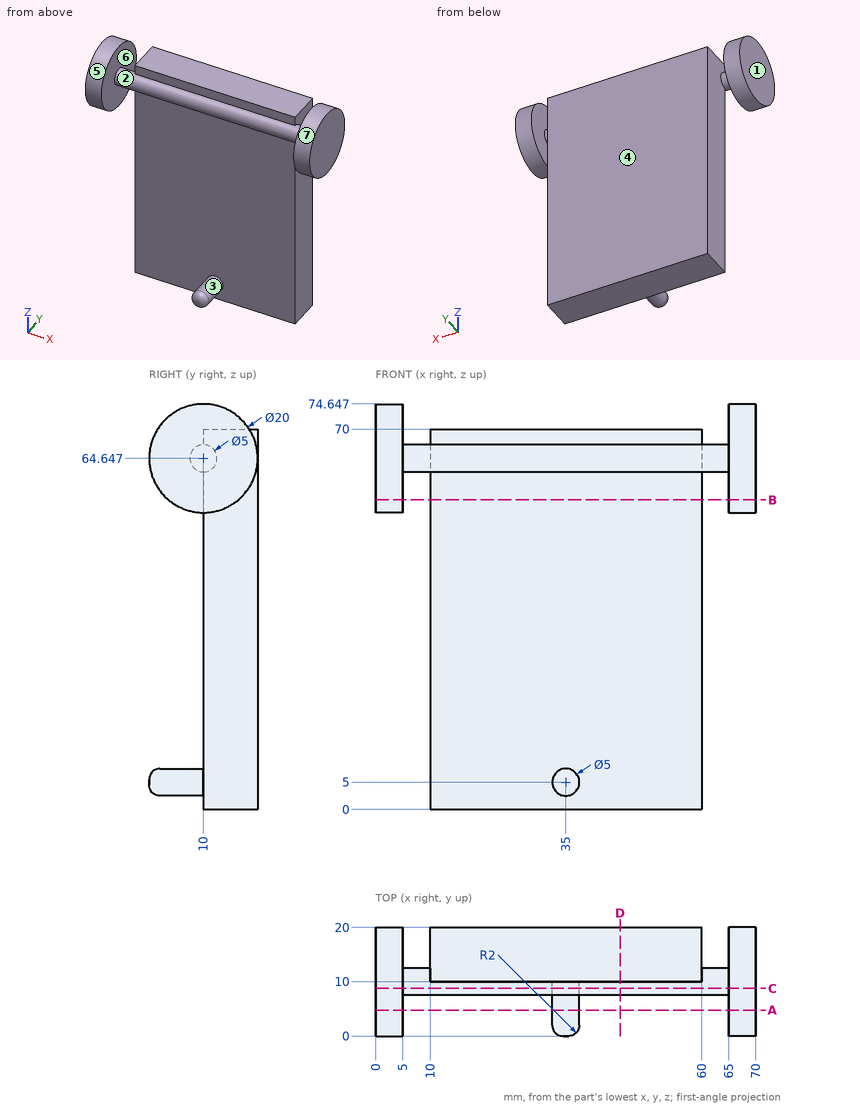
Geometry: see drawing. Coordinates: mm, zero at the bounding-box minimum. A direction names the side the tool comes from. Coordinates: 2 decimals unless noted, no trailing zeros. Order: outer loops, then holes, each group sorted by start corner. A loop starts at its lowest first (then second) coordinate and runs counter-clockwise, first axis right, second up. Notation, with made-up numbers: (38.5, 0.25) - (97.5, 0.25) arc R17 ccw to (97.5, 4.25) - close; hole circle Ø9 at (-35, 65). An arc over 180 degrees is marked (long way). Return JSON: item names as keys, results as strings.
Q1. First-contact query: pin 1 (0.9 mm diameter, centred on x = 44, z = 68.5, fed in from -Y); pin 2 (3 mm diameter, centred on y = 15, z = 34.5, fed in from +X); pin 3 (2 mm diameter, centred on x = 54.5, y = 9.5, fed in from +Z). Flat tips, straight axial feed; report the tip coordinate or a pass-through.
The answers:
{"pin 1": "stops at y = 10", "pin 2": "stops at x = 60", "pin 3": "stops at z = 70"}
Q2. Ray query, probe 1 along X at (y, z) = (13.5, 57); probe 2 along X at (y, z) = (13, 32.5); probe 3 along Y at (x, z) = (30, 64.5). Return the intervals inside material, ascending.
The answers:
{"probe 1": "x = 0 to 5, 10 to 60, 65 to 70", "probe 2": "x = 10 to 60", "probe 3": "y = 7.5 to 20"}
Q3. Cut plane C-C (y = 8.75). Return loops of the section in (x, z) (1 decimal), then the cut area to 3 significant figures.
The answers:
{"outline": "(0, 54.7) - (5, 54.7) - (5, 62.5) - (65, 62.5) - (65, 54.7) - (70, 54.7) - (70, 74.6) - (65, 74.6) - (65, 66.8) - (5, 66.8) - (5, 74.6) - (0, 74.6) - close; circle Ø5 at (35, 5)", "area": "478 mm2"}
Q4. Draft query along X for the marked faces 1, 2, 3 and 4. Return one class per face: +X half, -X half, draft (parallel to the pull), parting line (faces both ways), or undercut.
The answers:
{"face 1": "-X half", "face 2": "undercut", "face 3": "parting line", "face 4": "draft"}
Q5. Cut plane B-B (z = 57). Return loops of the section in (x, y), then the cut area to 3 significant figures.
The answers:
{"outline": "(0, 3.56) - (5, 3.56) - (5, 16.44) - (0, 16.44) - close; (10, 10) - (60, 10) - (60, 20) - (10, 20) - close; (65, 3.56) - (70, 3.56) - (70, 16.44) - (65, 16.44) - close", "area": "629 mm2"}
Q6. Cut plane A-A (y = 4.75). Return loops of the section in (x, z), then the cut area to 3 significant figures.
The answers:
{"outline": "(0, 56.14) - (5, 56.14) - (5, 73.16) - (0, 73.16) - close; circle Ø5 at (35, 5); (65, 56.14) - (70, 56.14) - (70, 73.16) - (65, 73.16) - close", "area": "190 mm2"}
Q7. Cut plane D-D (x = 45). Return loops of the section in (y, z), then the cut area to 3 significant figures.
The answers:
{"outline": "(10, 0) - (20, 0) - (20, 70) - (10, 70) - (10, 67.15) arc R2.5 ccw to (10, 62.15) - close", "area": "710 mm2"}
Q8. Access query for the marked faces 5, 6 and 7. Directions: +Z, -Z, +X, -X, +Y, -Y. A direction counts if a zero-diameter tool reaches every point of the face in a straight line with its end or side. Return the directions, or none.
The answers:
{"face 5": "-X", "face 6": "none", "face 7": "+X"}
